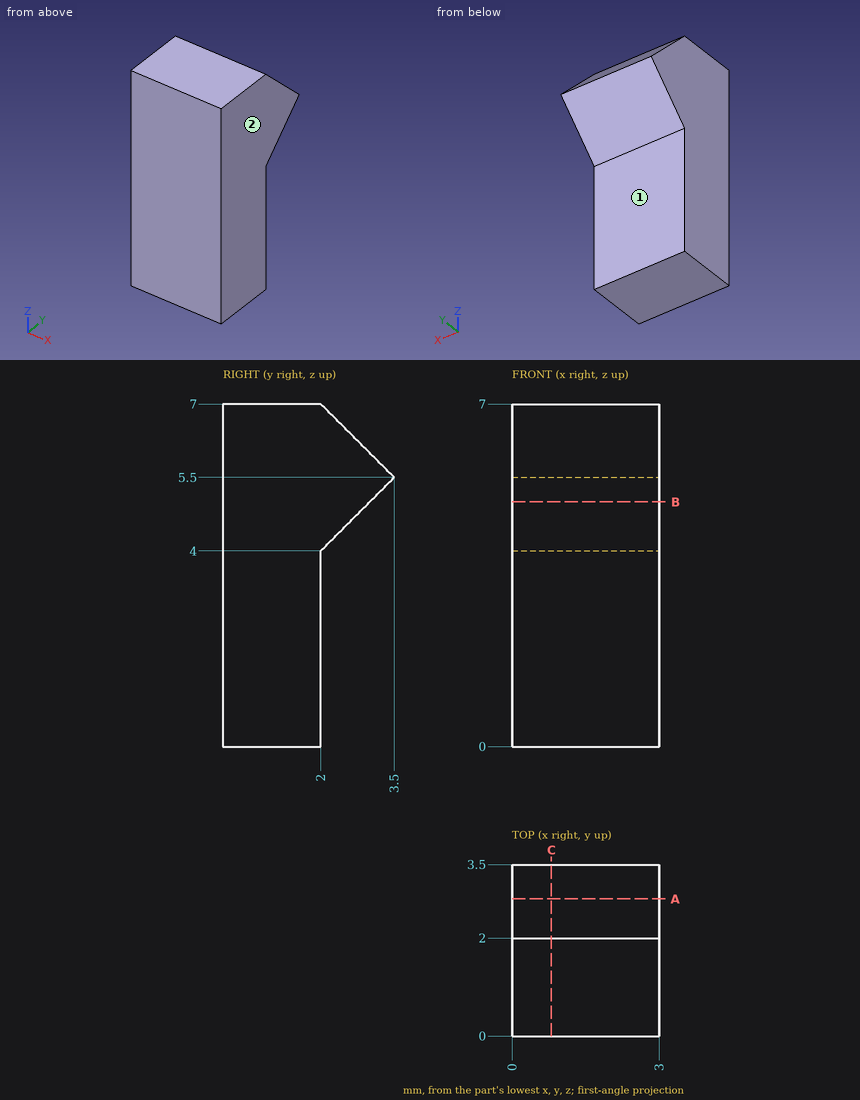
Could you check a few things on this drawing? It's one solid part, dimensions in mm from its lowest x, y, z. A direction names the side the tool comes from. Coordinates: 2 decimals unless noted, no trailing zeros. Order: outer loops, then holes, each group sorted by start corner. A loop starts at its lowest first (then second) coordinate and runs counter-clockwise, first axis right, second up.
1) Imagine slicing it at B-B on z = 5. List the corners of the cut face in (x, y) for me.
2) Will this pin go through, and if not, where does the flat tip stop? pin 1 (1.5 mm diameter, centred on x = 1.5, z = 2, fed in from +Y).
3) Which directions (+Z, -Z, +X, -X, +Y, -Y) give clear straight access to the entire face, cutting with the end or side of a thin tool? Please do the marked faces 1 and 2.
4) I need wall thicknesses on line 1 (Y direction, x = 0.85, z = 3.25); line 2 (Z direction, x = 0.75, y = 3.1); line 3 (Z direction, x = 2.2, y = 2.55). Which ranges of each line are inside material? Lowest first, please.
5) Imagine slicing it at C-C on x = 0.8. List the corners of the cut face in (y, z) for me.
6) Imagine slicing it at A-A on y = 2.8. List the corners of the cut face in (x, z) for me, and give its area (3 significant figures).
Response values:
1. outline: (0, 0) - (3, 0) - (3, 3) - (0, 3) - close
2. pin 1: stops at y = 2
3. face 1: -Z, +X, -X, +Y
3. face 2: +Z, -Z, +X, +Y, -Y
4. line 1: y = 0 to 2
4. line 2: z = 5.1 to 5.9
4. line 3: z = 4.55 to 6.45
5. outline: (0, 0) - (2, 0) - (2, 4) - (3.5, 5.5) - (2, 7) - (0, 7) - close
6. outline: (0, 4.8) - (3, 4.8) - (3, 6.2) - (0, 6.2) - close
6. area: 4.20 mm2
